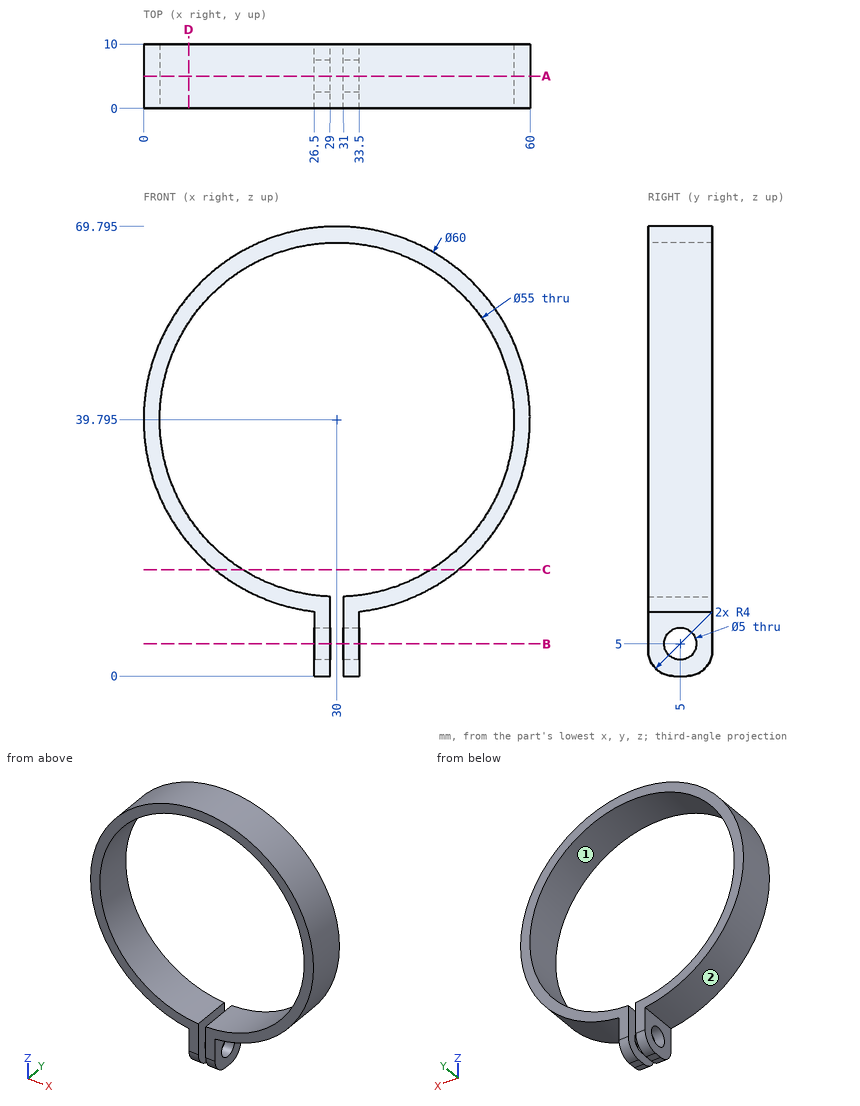
Can you work these out from the drawing? Everything is in mm from the part's minimum corner. Round coordinates to 2 decimals unless told otherwise and drop trailing zeros. Loops run counter-clockwise (first coordinate to the right, second up) from the corner with the lowest first, then second, coordinate; pieces in that order, holes last. Notation, with made-up numbers: (12, 65.5) - (18, 65.5) arc R18 ccw to (18, 71.5) - close; hole circle Ø1 at (-39.75, -11). An arc over 180 degrees is marked (long way). Write item = value, one per line. Start each with the question number.
(1) If we section it at B-B (z = 5): Please give me the cut outline in (x, y), and give its area (3 significant figures).
(2) If we section it at C-C (z = 16.5): Please give me the cut outline in (x, y).
(3) If we section it at A-A (y = 5): Please give me the cut outline in (x, z) (1 decimal), and give its area (3 significant figures).
(4) If I drill on probe 1 along X at (y, z) = (6.75, 9); probe 2 along Y at (x, z) = (32.8, 5); probe 3 along Z at (x, y) = (33, 6.75) (1 decimal), over which ranges is the centre line in solid material (lowest first)? Write a range as [from, to].
(5) If we section it at D-D (x = 7): Please give me the cut outline in (y, z).
(6) If we mould it in two halves opening along Z, with no side actions, what happens to the marked faces 1 and 2? For each: released by +Z, released by -Z, zero draft, split by the parting line, or undercut.
(7) For P1, Ø5, axis at y = 2.5, z = 6, coming from the -X side; P2, Ø5, axis at y = 5, z = 4.5, coming from the +X side; P3, Ø1.5, axis at y = 7.5, z = 46, coming from the +X side, each with a flat end and sliding along its axis, tell me the tip position at first contact or that it passes through.
Ans:
q1.outline = (26.5, 0) - (29, 0) - (29, 2.5) - (26.5, 2.5) - close; (26.5, 7.5) - (29, 7.5) - (29, 10) - (26.5, 10) - close; (31, 0) - (33.5, 0) - (33.5, 2.5) - (31, 2.5) - close; (31, 7.5) - (33.5, 7.5) - (33.5, 10) - (31, 10) - close
q1.area = 25.0 mm²
q2.outline = (11.1, 0) - (15.39, 0) - (15.39, 10) - (11.1, 10) - close; (44.61, 0) - (48.9, 0) - (48.9, 10) - (44.61, 10) - close
q3.outline = (26.5, 0) - (29, 0) - (29, 2.5) - (26.5, 2.5) - close; (26.5, 7.5) - (29, 7.5) - (29, 12.3) arc R27.5 cw (long way) to (31, 12.3) - (31, 7.5) - (33.5, 7.5) - (33.5, 10) arc R30 ccw (long way) to (26.5, 10) - close; (31, 0) - (33.5, 0) - (33.5, 2.5) - (31, 2.5) - close
q3.area = 471 mm²
q4.probe_1 = [26.5, 29], [31, 33.5]
q4.probe_2 = [0, 2.5], [7.5, 10]
q4.probe_3 = [0.1, 3.2], [6.8, 12.5], [67.1, 69.6]
q5.outline = (0, 20.53) - (10, 20.53) - (10, 24.72) - (0, 24.72) - close; (0, 54.87) - (10, 54.87) - (10, 59.06) - (0, 59.06) - close
q6.face_1 = undercut
q6.face_2 = split by the parting line
q7.P1 = 26.5
q7.P2 = 33.5
q7.P3 = 59.5
